from build123d import *

# Parameters (mm, degrees)
SKETCH_1_R      = 2.1
EXTRUDE_2_DEPTH = 2
FILLET_1_R      = 2


with BuildPart() as part:
    # ｽｹｯﾁ1 → ﾎﾞｽ - 押し出し2 (new body)
    with BuildSketch(Plane(origin=(0, 0, 0), x_dir=(1, 0, 0), z_dir=(0, 1, 0))):
        Polygon((36, 27), (-14, 27), (-22, 21), (-2.5, -5), (1.666666667, -5), (20, -5), (24.5, -5), (44, 21), align=None)
        with Locations(Location((0, 0, 0), (0, 0, 270))):
            Circle(SKETCH_1_R, mode=Mode.SUBTRACT)
        with BuildLine():
            ThreePointArc((20, -0.640312424), (19.9, 0), (20, 0.640312424))
            ThreePointArc((20, 0.640312424), (24.1, 0), (20, -0.640312424))
        make_face(mode=Mode.SUBTRACT)
        with Locations(Location((-15, 20, 0), (0, 0, 270))):
            Circle(SKETCH_1_R, mode=Mode.SUBTRACT)
        with Locations(Location((37, 20, 0), (0, 0, 270))):
            Circle(SKETCH_1_R, mode=Mode.SUBTRACT)
    extrude(amount=EXTRUDE_2_DEPTH)

    # ﾌｨﾚｯﾄ1
    fillet_1_edges = [part.edges().sort_by_distance(p)[0] for p in [
        (-22, 1, -21),
        (-14, 1, -27),
        (36, 1, -27),
        (44, 1, -21),
        (24.5, 1, 5),
        (-2.5, 1, 5),
    ]]
    fillet(fillet_1_edges, radius=FILLET_1_R)


solid = part.part
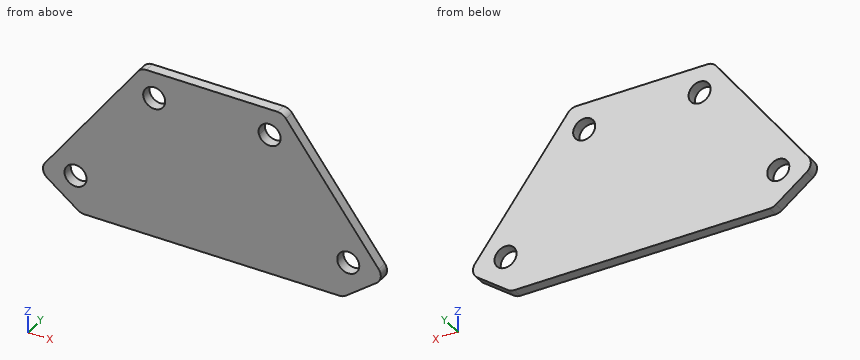
Geometry: final body of the model. Coordinates: model frame, mm. Round coordinates to 2 decimals unless told otherwise and drop trailing zeros. Order: outer loops, then holes, each group sorted by start corner. A loop starts at its lowest first (then second) coordinate and runs counter-clockwise, first axis right, second up.
Q1. Pin query (flat end, axial travel): pin 1 (3.5 mm diameter, centred on x = 37, z = -20, fed in from -Y). Return the tip coordinate at first contact, or that it passes through.
Result sheet:
pin 1: passes through
Q2. Section B-B, the plane x = 22. Output: boundary loops of the cut face in (y, z).
Result sheet:
outline: (0, -27) - (2, -27) - (2, -2.1) - (0, -2.1) - close; (0, 2.1) - (2, 2.1) - (2, 5) - (0, 5) - close
Q3. Section D-D, the plane z = -21. Output: boundary loops of the cut face in (x, y), and give its area (3 significant figures).
Result sheet:
outline: (-21.16, 0) - (-16.85, 0) - (-16.85, 2) - (-21.16, 2) - close; (-13.15, 0) - (35.15, 0) - (35.15, 2) - (-13.15, 2) - close; (38.85, 0) - (43.16, 0) - (43.16, 2) - (38.85, 2) - close
area: 114 mm2
Q4. Section C-C, the plane y = 1.1. Output: boundary loops of the cut face in (x, z).
Result sheet:
outline: (-20.8, -19.4) arc R2 ccw to (-20.4, -22.2) - (-14.53, -26.6) arc R2 ccw to (-13.33, -27) - (35.33, -27) arc R2 ccw to (36.53, -26.6) - (42.4, -22.2) arc R2 ccw to (42.8, -19.4) - (25.1, 4.2) arc R2 ccw to (23.5, 5) - (-1.5, 5) arc R2 ccw to (-3.1, 4.2) - close; hole circle Ø4.2 at (-15, -20); hole circle Ø4.2 at (0, 0); hole circle Ø4.2 at (22, 0); hole circle Ø4.2 at (37, -20)
Q5. Material intervals for probe 1 along X at (y, z) = (1.15, -20); probe 2 along X at (y, z) = (0.45, 0); probe 3 along Z at (x, y) = (22, 0.8), sorted ascending.
Result sheet:
probe 1: x = -21.11 to -17.1, -12.9 to 34.9, 39.1 to 43.11
probe 2: x = -6.25 to -2.1, 2.1 to 19.9, 24.1 to 28.25
probe 3: z = -27 to -2.1, 2.1 to 5
Q6. Section A-A, the plane z = 0. Output: boundary loops of the cut face in (x, y), and give its area (3 significant figures).
Result sheet:
outline: (-6.25, 0) - (-2.1, 0) - (-2.1, 2) - (-6.25, 2) - close; (2.1, 0) - (19.9, 0) - (19.9, 2) - (2.1, 2) - close; (24.1, 0) - (28.25, 0) - (28.25, 2) - (24.1, 2) - close
area: 52.2 mm2
